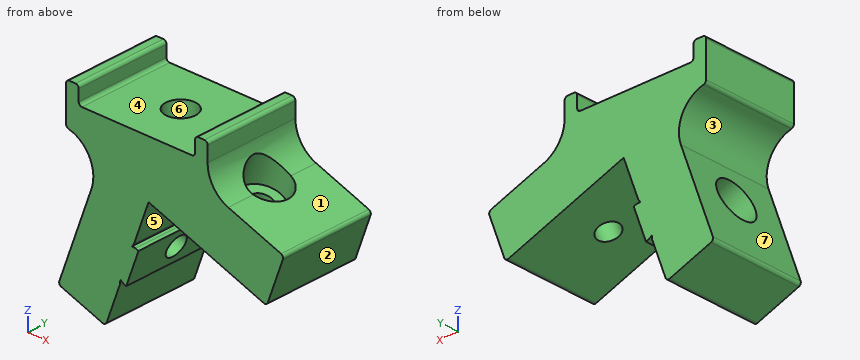
```python
from build123d import *

# Parameters (mm, degrees)
BOSS_EXTRUDE1_DEPTH                                 = 15
SKETCH4_R                                           = 2.35
CUT_EXTRUDE3_DEPTH                                  = 6
CBORE_FOR_M3_HEX_SOCKET_HEAD_CAP_SCREW1_D           = 3.4
CBORE_FOR_M3_HEX_SOCKET_HEAD_CAP_SCREW1_CBORE_D     = 6.5
CBORE_FOR_M3_HEX_SOCKET_HEAD_CAP_SCREW1_CBORE_DEPTH = 3.4
CUT_EXTRUDE4_DEPTH                                  = 40.36183231
SKETCH2_R                                           = 3.25
CUT_EXTRUDE5_DEPTH                                  = 42.264373258
FILLET4_R                                           = 5
FILLET5_R                                           = 5
FILLET6_R                                           = 0.5
FILLET7_R                                           = 0.5
FILLET8_R                                           = 0.5
FILLET9_R                                           = 0.5
FILLET10_R                                          = 0.5
FILLET11_R                                          = 0.5
FILLET12_R                                          = 0.5
FILLET13_R                                          = 0.5
FILLET14_R                                          = 0.5
FILLET15_R                                          = 0.5
FILLET16_R                                          = 0.5


with BuildPart() as part:
    # Sketch1 → Boss-Extrude1 (new body)
    with BuildSketch(Plane(origin=(0, 0, 0), x_dir=(1, 0, 0), z_dir=(0, 1, 0))):
        Polygon((-23.760232958, -5.596615827), (-31.459597373, 15.557214047), (-23.942056406, 18.293375193), (-17.10165354, -0.500477222), (1.692198876, 6.339925644), (4.428360022, -1.177615322), (-7.712744083, -5.596615827), align=None)
        Polygon((-20.650889023, 11.882391084), (-21.496612382, 11.574572955), (-19.547097565, 6.218325016), (-18.701374206, 6.526143145), align=None)
        Polygon((-18.962744083, -5.596615827), (-23.760232958, -5.596615827), (-30.212744083, -5.596615827), (-30.212744083, -11.939309749), (-28.212744083, -11.939309749), (-28.212744083, -9.189582126), (-9.712744083, -9.189582126), (-9.712744083, -11.939309749), (-7.712744083, -11.939309749), (-7.712744083, -5.596615827), align=None)
    extrude(amount=BOSS_EXTRUDE1_DEPTH)

    # Sketch4 → Cut-Extrude3 (cut)
    with BuildSketch(Plane(origin=(0, 0, 9.189582126), x_dir=(-1, 0, 0), z_dir=(0, 0, -1))):
        with Locations((18.962744083, 7.5)):
            Circle(SKETCH4_R)
    extrude(amount=CUT_EXTRUDE3_DEPTH, mode=Mode.SUBTRACT)

    # CBORE for M3 Hex Socket Head Cap Screw1 (through all)
    with Locations(Plane(origin=(-22.779531346, 0, 8.291071361), x_dir=(0.34202014332566366, 0, 0.9396926207859102), z_dir=(-0.9396926207859103, 0, 0.3420201433256637))):
        with Locations((-15.378815242, 7.5)):
            CounterBoreHole(CBORE_FOR_M3_HEX_SOCKET_HEAD_CAP_SCREW1_D / 2, CBORE_FOR_M3_HEX_SOCKET_HEAD_CAP_SCREW1_CBORE_D / 2, CBORE_FOR_M3_HEX_SOCKET_HEAD_CAP_SCREW1_CBORE_DEPTH)

    # Sketch10 → CBORE for M3 Hex Socket Head Cap Screw2 (revolve, cut)
    with BuildSketch(Plane(origin=(-4.968566186, 7.5, 4.597816755), x_dir=(0.9396926207859094, 0, -0.34202014332566627), z_dir=(0, 1, 0))):
        Polygon((0, 0), (0, 30.571150439), (1.7, 30.571150439), (1.7, 3.4), (3.25, 3.4), (3.25, 0), align=None)
    revolve(axis=Axis((-2.796738275, 7.5, 10.564864897), (-0.34202014332566627, 0, -0.9396926207859094)), mode=Mode.SUBTRACT)

    # Sketch11 → Cut-Extrude4 (cut, through all)
    with BuildSketch(Plane(origin=(0, 15, 0), x_dir=(1, 0, 0), z_dir=(0, 1, 0))):
        Polygon((-21.633420439, 11.950450003), (-21.589873913, 11.374572955), (-21.120735333, 11.711381012), (-21.496612382, 11.574572955), align=None)
    cut_extrude4 = extrude(amount=-CUT_EXTRUDE4_DEPTH, mode=Mode.SUBTRACT)

    # Mirror1: Cut-Extrude4 across plane
    add(cut_extrude4.mirror(Plane(origin=(-5.259864593, 0, -14.4513592), x_dir=(0.9396926207859102, 0, -0.3420201433256638), z_dir=(-0.3420201433256638, 0, -0.9396926207859102))), mode=Mode.SUBTRACT)

    # Sketch2 → Cut-Extrude5 (cut, through all)
    with BuildSketch(Plane(origin=(0.896497987, 0, 2.463107975), x_dir=(0.9396926207859094, 0, -0.34202014332566627), z_dir=(0.34202014332566627, 0, 0.9396926207859094))):
        with Locations((-6.241470926, 7.5)):
            Circle(SKETCH2_R)
    extrude(amount=CUT_EXTRUDE5_DEPTH, mode=Mode.SUBTRACT)

    # Fillet4
    # the kernel refuses this fillet: 5 mm, written as the material it adds along each edge
    with BuildSketch(Plane(origin=(-23.760232958, 0, 5.596615827), x_dir=(-0.34202014332566355, 0, -0.9396926207859103), z_dir=(0, 1, 0))) as fillet4_piece_1:
        with BuildLine():
            CenterArc((7.092503292, 5), FILLET4_R, 167.720815182, 102.279184818)
            Line((2.20688878, 6.06337709), (2.10917649, 6.084644632))
            ThreePointArc((2.10917649, 6.084644632), (1.009475128, 3.065890559), (-0.093969262, 0.034202014))
            Line((-0.093969262, 0.034202014), (0, -0.1))
            Line((0, -0.1), (7.092503292, -0.1))
            Line((7.092503292, -0.1), (7.092503292, 0))
        make_face()
    extrude(amount=15)

    # Fillet5
    # the kernel refuses this fillet: 5 mm, written as the material it adds along each edge
    with BuildSketch(Plane(origin=(-7.712744083, 0.173725541, 5.596615827), x_dir=(0, 0, 1), z_dir=(0, 1, 0))) as fillet5_piece_1_section:
        with BuildLine():
            CenterArc((FILLET5_R * 0.70020753821, FILLET5_R), FILLET5_R, 200, 70)
            Line((-FILLET5_R * 0.239485082576, FILLET5_R * 0.657979856674), (0, 0))
            Line((0, 0), (FILLET5_R * 0.70020753821, 0))
        make_face()
    fillet5_piece_1 = extrude(amount=14.826274459, mode=Mode.PRIVATE)
    fillet5_piece_1 = fillet5_piece_1 - Plane(origin=(-4.162007445, 7.5, 6.813818681), x_dir=(0.9396926207859094, 0, -0.34202014332566627), z_dir=(-0.34202014332566627, 0, -0.9396926207859094)) * Cylinder(3.25, 44, mode=Mode.PRIVATE)
    add(fillet5_piece_1)
    with BuildSketch(Plane(origin=(-7.712744083, 0, 5.596615827), x_dir=(0, 0, 1), z_dir=(0, 1, 0))) as fillet5_piece_2_section:
        with BuildLine():
            CenterArc((FILLET5_R * 0.70020753821, FILLET5_R), FILLET5_R, 200, 70)
            Line((-FILLET5_R * 0.239485082576, FILLET5_R * 0.657979856674), (0, 0))
            Line((0, 0), (FILLET5_R * 0.70020753821, 0))
        make_face()
    fillet5_piece_2 = extrude(amount=14.826274459, mode=Mode.PRIVATE)
    fillet5_piece_2 = fillet5_piece_2 - Plane(origin=(-4.162007445, 7.5, 6.813818681), x_dir=(0.9396926207859094, 0, -0.34202014332566627), z_dir=(-0.34202014332566627, 0, -0.9396926207859094)) * Cylinder(3.25, 44, mode=Mode.PRIVATE)
    add(fillet5_piece_2)

    # Fillet6
    fillet6_edges = [part.edges().sort_by_distance(p)[0] for p in [
        (-28.212744083, 7.5, 9.189582126),
    ]]
    fillet(fillet6_edges, radius=FILLET6_R)

    # Fillet7
    fillet7_edges = [part.edges().sort_by_distance(p)[0] for p in [
        (-9.712744083, 7.5, 9.189582126),
    ]]
    fillet(fillet7_edges, radius=FILLET7_R)

    # Fillet8
    fillet8_edges = [part.edges().sort_by_distance(p)[0] for p in [
        (-28.212744083, 7.5, 11.939309749),
    ]]
    fillet(fillet8_edges, radius=FILLET8_R)

    # Fillet9
    fillet9_edges = [part.edges().sort_by_distance(p)[0] for p in [
        (-9.712744083, 7.5, 11.939309749),
    ]]
    fillet(fillet9_edges, radius=FILLET9_R)

    # Fillet10
    fillet10_edges = [part.edges().sort_by_distance(p)[0] for p in [
        (-30.212744083, 7.5, 11.939309749),
    ]]
    fillet(fillet10_edges, radius=FILLET10_R)

    # Fillet11
    fillet11_edges = [part.edges().sort_by_distance(p)[0] for p in [
        (-7.712744083, 7.5, 11.939309749),
    ]]
    fillet(fillet11_edges, radius=FILLET11_R)

    # Fillet12
    fillet12_edges = [part.edges().sort_by_distance(p)[0] for p in [
        (4.428360022, 7.5, 1.177615322),
    ]]
    fillet(fillet12_edges, radius=FILLET12_R)

    # Fillet13
    fillet13_edges = [part.edges().sort_by_distance(p)[0] for p in [
        (1.692198876, 7.5, -6.339925644),
    ]]
    fillet(fillet13_edges, radius=FILLET13_R)

    # Fillet14
    fillet14_edges = [part.edges().sort_by_distance(p)[0] for p in [
        (-23.942056406, 7.5, -18.293375193),
    ]]
    fillet(fillet14_edges, radius=FILLET14_R)

    # Fillet15
    fillet15_edges = [part.edges().sort_by_distance(p)[0] for p in [
        (-31.459597373, 7.5, -15.557214047),
    ]]
    fillet(fillet15_edges, radius=FILLET15_R)

    # Fillet16
    fillet16_edges = [part.edges().sort_by_distance(p)[0] for p in [
        (-30.212744083, 7.5, 5.596615827),
    ]]
    fillet(fillet16_edges, radius=FILLET16_R)


solid = part.part
```
Model file for the job. Use its own axes, mm. Face numbers are marked on the shaded views. A direction names the side the tool comes from. Give positions to 0.01 mm unless a question says otherwise; leave off trailing zeros. Loops run counter-clockwise (first coordinate to the right, second up) from the corner with the lowest first, then second, coordinate; pieces in that order, holes last. Notation, with made-up numbers: (-24, 78.5) - (-12, 78.5) arc R14 ccw to (-12, 104.5) - close; hole circle Ø3 at (2.25, -9). An arc over 180 degrees is marked (long way). One line per item, written item: value. Start each with the question number.
1. Slice it at D-D (z = -14). List the corners of the cut face in (x, y), plus the area to 3 significant figures.
2. Pin check, flat tips, straight feed: pin 1 (1.9 mm diameter, centred on y = 10.5, z = 11, fed in from -X); pin 2 (6 mm diameter, centred on x = -20.5, y = 4.5, fed in from +Z); pin 3 (0.7 mm diameter, centred on y = 8, z = 10.5, fed in from +X); pin 4 (10 mm diameter, centred on x = -7, z = -10.5, fed in from +Y). Stop position of each tip, or through.
3. Pull direction Z, two halves, no side cores. Call the marked faces 1, 2 and 3: pulls with the +Z half, pulls with the -Z half, needs draft (parallel to the pull), parting line crosses it, or undercut.
4. Slice it at B-B (x = -17.5). List the corners of the cut face in (y, z).
5. Slice it at C-C (y = 7.5). Give the number of separate pieces and of enclosed holes in the cut face, plus the area to 3 significant figures.
6. Probe L1, parallel to Y at x = -25, z = -5; L2, parallel to Y at x = -27.5, z = -9; L3, parallel to Z at x = -16.5, y = 11.5. List the from-to ranges inside material, lowest first. Write a range as from..to.
7. Which spindle directions (+Z, -Z, +X, -X, +Y, -Y) get a long thin tool onto all of the face, cutting with end or side? Do the marked faces 4, 5, 6 and 7. Say none if no direction does.
Solution:
1. outline: (-30.89, 0) - (-22.38, 0) - (-22.38, 15) - (-30.89, 15) - close
1. area: 128 mm^2
2. pin 1: stops at x = -30.21
2. pin 2: stops at z = 9.19
2. pin 3: stops at x = -7.71
2. pin 4: passes through
3. face 1: pulls with the +Z half
3. face 2: pulls with the -Z half
3. face 3: undercut
4. outline: (0, -0.59) - (15, -0.59) - (15, 9.19) - (9.34, 9.19) - (9.34, 3.19) - (5.66, 3.19) - (5.66, 9.19) - (0, 9.19) - close
5. separate pieces: 3
5. enclosed holes: 0
5. area: 344 mm^2
6. L1: y = 0..5.05, 9.95..15
6. L2: y = 0..5.4, 9.6..15
6. L3: z = 0.28..9.19
7. face 4: +Z, +Y, -Y
7. face 5: +Y, -Y
7. face 6: +Z
7. face 7: -X, +Y, -Y
